Geometry: see drawing. Coordinates: mm, zero at the bounding-box minimum. Coordinates: 2 decimals unless noted, no trailing zeros. Order: outer loops, then holes, each group sorted by start corner. A loop starts at its lowest first (then second) coordinate and runs counter-clockwise, first axis right, second up. Notation, with made-up numbers: M -28,0.25 L 22,0.25 A26 ccw 22,32.25 Z; hole C 48,46.5 d11. An arc over 180 degrees is marked long. One line per item, written item: value.
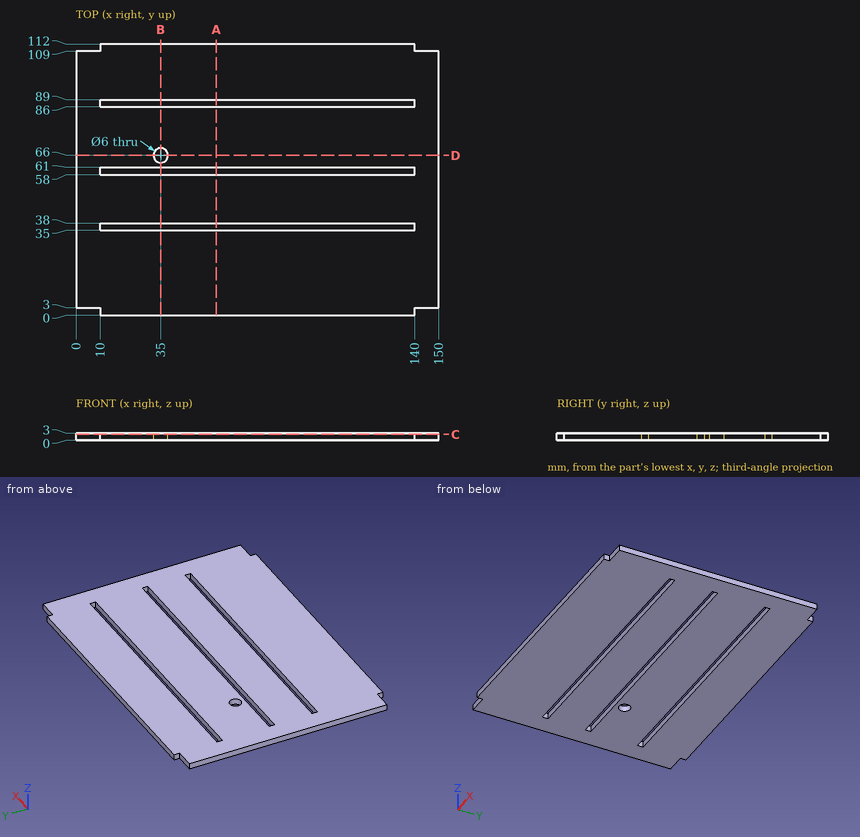
(1) Cut plane D-D on y = 66. Output: boundary loops of the cut face in (x, z).
Data:
outline: M 0,0 L 32,0 L 32,3 L 0,3 Z; M 38,0 L 150,0 L 150,3 L 38,3 Z
(2) Cut plane B-B on x = 35. Output: boundary loops of the cut face in (y, z).
Data:
outline: M 0,0 L 35,0 L 35,3 L 0,3 Z; M 38,0 L 58,0 L 58,3 L 38,3 Z; M 61,0 L 63,0 L 63,3 L 61,3 Z; M 69,0 L 86,0 L 86,3 L 69,3 Z; M 89,0 L 112,0 L 112,3 L 89,3 Z
(3) Cut plane C-C on z = 2.4. Output: boundary loops of the cut face in (x, y), plus the area to 3 significant figures.
Data:
outline: M 0,3 L 10,3 L 10,0 L 140,0 L 140,3 L 150,3 L 150,109 L 140,109 L 140,112 L 10,112 L 10,109 L 0,109 Z; hole M 10,35 L 140,35 L 140,38 L 10,38 Z; hole M 10,58 L 140,58 L 140,61 L 10,61 Z; hole M 10,86 L 140,86 L 140,89 L 10,89 Z; hole C 35,66 d6
area: 15,500 mm2
(4) First-contact query: pin 1 (5.5 mm diameter, centred on x = 35, y = 66, fed in from -Z); pin 2 (1.5 mm diameter, centred on y = 1, z = 2, fed in from +X); pin 3 (0.9 mm diameter, centred on y = 110.5, z = 1.5, fed in from -X); pin 4 (0.9 mm diameter, centred on x = 144, z = 2, fed in from +Y). Flat tips, straight axial feed; report the tip coordinate or a pass-through.
Data:
pin 1: passes through
pin 2: stops at x = 140
pin 3: stops at x = 10
pin 4: stops at y = 109
(5) Cut plane A-A on x = 58. Output: boundary loops of the cut face in (y, z), plus the area to 3 significant figures.
Data:
outline: M 0,0 L 35,0 L 35,3 L 0,3 Z; M 38,0 L 58,0 L 58,3 L 38,3 Z; M 61,0 L 86,0 L 86,3 L 61,3 Z; M 89,0 L 112,0 L 112,3 L 89,3 Z
area: 309 mm2
(6) Ray query, line 1 (Y direction, x = 35, z = 1.6); line 2 (Y direction, x = 22.5, z = 0.4); line 3 (Y direction, x = 9.5, z = 1.75). Return the intervals inside material, ascending. Write a range as from..to.
Data:
line 1: y = 0..35, 38..58, 61..63, 69..86, 89..112
line 2: y = 0..35, 38..58, 61..86, 89..112
line 3: y = 3..109
